Part model, mm, in its own coordinate system. Face numbers are marked on the shaded views. Coordinates: 2 decimals unless noted, no trailing zeros. Write each loop counter-clockwise with the first axis right and the second up, starting at its lowest first coordinate (ties: lowest second). Pieces come first, ordered by that corner, then holes. Notation, with made-up numbers: (65, 75) - (92, 75) arc R25 cw to (92, 109) - close; hole circle Ø8 at (55, 21). An arc over 180 degrees is marked (long way). Write each question's results on one line, items separated by ' | '.
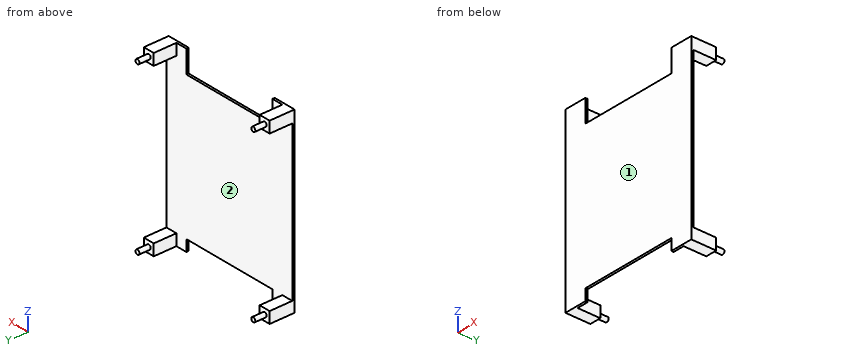
Autodesk Inventor part; units mm, degrees
ref_plane "YZ Plane" through (0, 0, 0) normal (1, 0, 0) x (0, 1, 0)
ref_plane "XZ Plane" through (0, 0, 0) normal (0, 1, 0) x (-1, 0, 0)
ref_plane "XY Plane" through (0, 0, 0) normal (0, 0, 1) x (1, 0, 0)
sketch "Sketch1" plane through (0, 0, 0) normal (0, 1, 0) x (-1, 0, 0)
  line L0 (0, 0) -> (53.34, 0)
  line L1 (53.34, 0) -> (53.34, -68.58)
  line L2 (53.34, -68.58) -> (0, -68.58)
  line L3 (0, -68.58) -> (0, 0)
  line L4 (53.34, -66) -> (0, -66) construction
  circle A0 centre (7.62, -66) radius 1.5
  circle A1 centre (35.56, -66) radius 1.5
  circle A2 centre (2.5, -14) radius 1.5
  line L5 (-5, -73.58) -> (58.34, -73.58)
  line L6 (58.34, -73.58) -> (58.34, 5)
  line L7 (58.34, 5) -> (-5, 5)
  line L8 (-5, 5) -> (-5, -73.58)
  dimension "d0" = 68.58
  dimension "d1" = 53.34
  dimension "d2" = 2.58
  dimension "d3" = 3
  dimension "d4" = 7.62
  dimension "d5" = 3
  dimension "d6" = 35.56
  dimension "d8" = 3
  dimension "d9" = 14
  dimension "d10" = 2.5
  dimension "d46" = 5
extrude "Extrusion4" add sketch "Sketch1" along normal blind 1 contours L0 L1 L2 L3 | A0 | A1 | A2 | L8 L7 L6 L5
sketch "Sketch5" plane through (0, 1, 0) normal (0, 1, 0) x (1, 0, 0)
  line L0 (5, -5) -> (0, -5)
  line L1 (0, -5) -> (0, 0)
  line L2 (0, 0) -> (5, 0)
  line L3 (5, 0) -> (5, -5)
  dimension "d49" = 5
  dimension "d50" = 5
extrude "Extrusion5" add sketch "Sketch5" along normal blind 10
ref_plane "Work Plane2" through (-26.67, 0, 5) normal (1, 0, 0) x (0, 0, -1)
mirror "Mirror2" about plane through (-26.67, 0, 5) normal (1, 0, 0) of "Extrusion5"
ref_plane "Work Plane3" through (-58.34, 0, -34.29) normal (0, 0, 1) x (1, 0, 0)
mirror "Mirror3" about plane through (-58.34, 0, -34.29) normal (0, 0, 1) of "Extrusion5", "Mirror2"
sketch "Sketch7" plane through (0, 11, 0) normal (0, 1, 0) x (1, 0, 0)
  line L0 (0, 0) -> (0, -5)
  line L1 (0, -5) -> (5, -5)
  line L2 (5, -5) -> (5, 0)
  line L3 (5, 0) -> (0, 0)
  circle A0 centre (2.5, -2.5) radius 0.995
  dimension "d53" = 5
  dimension "d54" = 1.99
extrude "Extrusion8" add sketch "Sketch7" along normal blind 5 contours A0
mirror "Mirror10" about plane through (-26.67, 0, 5) normal (1, 0, 0) of "Extrusion8"
mirror "Mirror11" about plane through (-58.34, 0, -34.29) normal (0, 0, 1) of "Extrusion8", "Mirror10"
sketch "Sketch8" plane through (0, 1, 0) normal (0, 1, 0) x (1, 0, 0)
  line L0 (-53.34, 73.58) -> (-53.34, 68.58)
  line L1 (-53.34, 68.58) -> (-58.34, 68.58)
  line L2 (-58.34, 68.58) -> (-58.34, 0)
  line L3 (-58.34, 0) -> (-53.34, 0)
  line L4 (-53.34, 0) -> (-53.34, -5)
  line L5 (-53.34, -5) -> (0, -5)
  line L6 (0, -5) -> (0, 0)
  line L7 (0, 0) -> (5, 0)
  line L8 (5, 0) -> (5, 68.58)
  line L9 (5, 68.58) -> (0, 68.58)
  line L10 (0, 68.58) -> (0, 73.58)
  line L11 (0, 73.58) -> (-53.34, 73.58)
  line L12 (-58.34, -5) -> (5, -5)
  line L13 (-48.34, 5) -> (-5, 5)
  line L14 (-5, 5) -> (-5, -5)
  line L15 (-5, -5) -> (-48.34, -5)
  line L16 (-48.34, -5) -> (-48.34, 5)
  line L17 (5, -5) -> (5, 73.58)
  line L18 (5, 73.58) -> (-58.34, 73.58)
  line L19 (-48.34, 73.58) -> (-5, 73.58)
  line L20 (-5, 73.58) -> (-5, 68.58)
  line L21 (-5, 68.58) -> (-48.34, 68.58)
  line L22 (-48.34, 68.58) -> (-48.34, 73.58)
  dimension "d64" = 53.34
  dimension "d65" = 43.34
  dimension "d66" = 5
  dimension "d69" = 78.58
  dimension "d72" = 10
  dimension "d73" = 5
  dimension "d74" = 5
extrude "Extrusion9" cut sketch "Sketch8" against normal blind 1 contours L11 L20 L21 L22 | L16 L13 L14 L5
properties part number "boardtable2"
(1) Flat gauge pins, fed straight in: P1, Ø0.5, axis at x = -22, y = 0.5, coming from the +Z side; P2, Ø0.5, axis at x = -34.5, y = 0.5, coming from the -Z side. Where does each tip first touch, or does it go through?
Return value:
P1: stops at z = -5 | P2: stops at z = -68.58
(2) Wall check: line 1 (Z direction, x = 1.5, y = 10.75); line 2 (Y direction, x = -1.5, z = -58); line 3 (Z direction, x = -55, y = 14.25). Give the ranges that are in metal, low to high. Write a range as from..to.
Return value:
line 1: z = -73.58..-68.58, 0..5 | line 2: y = 0..1 | line 3: z = -71.61..-70.55, 1.97..3.03
(3) Two-plate mould, pull along Z, no slides. Class the marked faces 1 and 2: released by +Z, released by -Z, zero draft, split by the parting line, or undercut.
Return value:
face 1: zero draft | face 2: undercut
(4) Saw through at D-D on y = 13.75. Write the cut outline in (x, z) (3 decimals).
Return value:
outline: circle Ø1.99 at (-55.84, -71.08); circle Ø1.99 at (-55.84, 2.5); circle Ø1.99 at (2.5, -71.08); circle Ø1.99 at (2.5, 2.5)
(5) Saw through at B-B on x = 2.5. Write the cut outline in (y, z) (3 decimals), then the cut area to 3 significant figures.
Return value:
outline: (0, -73.58) - (11, -73.58) - (11, -72.075) - (16, -72.075) - (16, -70.085) - (11, -70.085) - (11, -68.58) - (1, -68.58) - (1, 0) - (11, 0) - (11, 1.505) - (16, 1.505) - (16, 3.495) - (11, 3.495) - (11, 5) - (0, 5) - close | area: 198 mm^2
(6) Saw through at A-A on z = 2.5. Write the cut outline in (x, y) (3 decimals).
Return value:
outline: (-58.34, 0) - (-48.34, 0) - (-48.34, 1) - (-53.34, 1) - (-53.34, 11) - (-54.845, 11) - (-54.845, 16) - (-56.835, 16) - (-56.835, 11) - (-58.34, 11) - close; (-5, 0) - (5, 0) - (5, 11) - (3.495, 11) - (3.495, 16) - (1.505, 16) - (1.505, 11) - (0, 11) - (0, 1) - (-5, 1) - close
(7) Saw through at C-C on y = 6. Write the cut outline in (x, z), then the cut area to 3 significant figures.
Return value:
outline: (-58.34, -73.58) - (-53.34, -73.58) - (-53.34, -68.58) - (-58.34, -68.58) - close; (-58.34, 0) - (-53.34, 0) - (-53.34, 5) - (-58.34, 5) - close; (0, -73.58) - (5, -73.58) - (5, -68.58) - (0, -68.58) - close; (0, 0) - (5, 0) - (5, 5) - (0, 5) - close | area: 100 mm^2
